from build123d import *

# Parameters (mm, degrees)
BOSS_EXTRUDE1_DEPTH                            = 3
CSK_FOR_M3_FLAT_HEAD_MACHINE_SCREW1_AT_2_COUNT = 2
CSK_FOR_M3_FLAT_HEAD_MACHINE_SCREW1_AT_2_PITCH = 71.314927951
CSK_FOR_M3_FLAT_HEAD_MACHINE_SCREW1_AT_3_COUNT = 2
CSK_FOR_M3_FLAT_HEAD_MACHINE_SCREW1_AT_3_PITCH = 7.071067812
CSK_FOR_M3_FLAT_HEAD_MACHINE_SCREW1_AT_4_COUNT = 2
CSK_FOR_M3_FLAT_HEAD_MACHINE_SCREW1_AT_4_PITCH = 123.124200131
CSK_FOR_M3_FLAT_HEAD_MACHINE_SCREW1_AT_5_COUNT = 2
CSK_FOR_M3_FLAT_HEAD_MACHINE_SCREW1_AT_5_PITCH = 117.544882759


with BuildPart() as part:
    # Sketch1 → Boss-Extrude1 (new body)
    with BuildSketch(Plane(origin=(0, 0, 0), x_dir=(1, 0, 0), z_dir=(0, 1, 0))):
        with BuildLine():
            Line((12, 68.963758598), (12, -68.802405773))
            Line((12, -68.802405773), (-53.528576558, -45.107554707))
            ThreePointArc((-53.528576558, -45.107554707), (-60.697790714, 34.868011163), (12, 68.963758598))
        make_face()
    extrude(amount=BOSS_EXTRUDE1_DEPTH)

    # Sketch4 → CSK for M3 Flat Head Machine Screw1 (revolve, cut)
    with BuildSketch(Plane(origin=(15, 3, 59), x_dir=(0, 0, 1), z_dir=(1, 0, 0))):
        Polygon((0, 0), (0, 3), (1.7, 3), (1.7, 1.65), (3.35, 0), align=None)
    csk_for_m3_flat_head_machine_screw1 = revolve(axis=Axis((15, 9.35, 59), (0, -1, 0)), mode=Mode.SUBTRACT)

    # CSK for M3 Flat Head Machine Screw1 at 2: CSK for M3 Flat Head Machine Screw1 ×2
    with Locations(*[Vector(-0.9512076756694684, 0, -0.30855138591081943) * (i * CSK_FOR_M3_FLAT_HEAD_MACHINE_SCREW1_AT_2_PITCH) for i in range(1, CSK_FOR_M3_FLAT_HEAD_MACHINE_SCREW1_AT_2_COUNT)]):
        add(csk_for_m3_flat_head_machine_screw1, mode=Mode.SUBTRACT)

    # CSK for M3 Flat Head Machine Screw1 at 3: CSK for M3 Flat Head Machine Screw1 ×2
    with Locations(*[Vector(-0.9899494936611665, 0, 0.14142135623730978) * (i * CSK_FOR_M3_FLAT_HEAD_MACHINE_SCREW1_AT_3_PITCH) for i in range(1, CSK_FOR_M3_FLAT_HEAD_MACHINE_SCREW1_AT_3_COUNT)]):
        add(csk_for_m3_flat_head_machine_screw1, mode=Mode.SUBTRACT)

    # CSK for M3 Flat Head Machine Screw1 at 4: CSK for M3 Flat Head Machine Screw1 ×2
    with Locations(*[Vector(-0.053450585626457235, 0, -0.9985704957068323) * (i * CSK_FOR_M3_FLAT_HEAD_MACHINE_SCREW1_AT_4_PITCH) for i in range(1, CSK_FOR_M3_FLAT_HEAD_MACHINE_SCREW1_AT_4_COUNT)]):
        add(csk_for_m3_flat_head_machine_screw1, mode=Mode.SUBTRACT)

    # CSK for M3 Flat Head Machine Screw1 at 5: CSK for M3 Flat Head Machine Screw1 ×2
    with Locations(*[Vector(-0.5771013187861944, 0, -0.8166725585295709) * (i * CSK_FOR_M3_FLAT_HEAD_MACHINE_SCREW1_AT_5_PITCH) for i in range(1, CSK_FOR_M3_FLAT_HEAD_MACHINE_SCREW1_AT_5_COUNT)]):
        add(csk_for_m3_flat_head_machine_screw1, mode=Mode.SUBTRACT)


solid = part.part
The listing builds one solid part. Answer for the finished solid, in the listing's coordinates (mm). Coordinates: 2 decimals unless noted, no trailing zeros. Loops run counter-clockwise (first coordinate to the right, second up) from the corner with the lowest first, then second, coordinate; pieces in that order, holes last.
1) Determine the mould class of faces 1 (the face through (-53.98, 0.68, -38.25)), 2 (the face through (-19, 0, -2)), 3 (the face through (12, 1, -1)) for opening direction X: pulls with the +X half, pulls with the -X half, needs draft (parallel to the pull), parting line crosses it, or undercut.
2) Find section C-C on z = -21. Write down the section's boundary in (x, y).
3) Find section A-A on y = 0.7. Write down the section's boundary in (x, z).
4) Flat-ended cylindrical pins translate along their axes: pin 1 Ø3 at (x, z) = (8.42, -63.95) entering from -Y; pin 2 Ø4.5 at (x, z) = (-52.84, 37) entering from +Y; pin 3 Ø1.5 at (x, y) = (2.5, 2) entering from -Z. Find the tip coordinate at first contact, or state that the pin passes through.
5) Find the intervals of material crossed by L1, parallel to Z at x = 8, y = 0.9; L2, parallel to X at y = 0.8, z = -1.5; L3, parallel to X at y = 1.4, z = 36, in increasing order.
6) Find section B-B on x = -28.5. Write down the section's boundary in (y, z), then the cut area to 3 significant figures.
Values:
1. face 1: undercut
1. face 2: needs draft
1. face 3: pulls with the +X half
2. outline: (-66.78, 0) - (12, 0) - (12, 3) - (-66.78, 3) - close
3. outline: (-53.53, 45.11) arc R70 ccw to (12, -68.96) - (12, 68.8) - close; hole circle Ø3.4 at (-52.84, -37); hole circle Ø3.4 at (-52.84, 37); hole circle Ø3.4 at (8, 60); hole circle Ø3.4 at (8.42, -63.95)
4. pin 1: passes through
4. pin 2: stops at y = 1.91
4. pin 3: stops at z = -69.98
5. L1: z = -69.54 to -65.6, -62.3 to 58.3, 61.7 to 67.36
5. L2: x = -69.98 to 12
5. L3: x = -60.03 to -54.27, -51.4 to 12
6. outline: (0, -63.94) - (3, -63.94) - (3, 54.16) - (0, 54.16) - close
6. area: 354 mm2
